Source: CAD feature listing. Evaluate the final solid. Frame: model axes, mm. Face numbers are marked on the shaded views. A direction names the side the tool comes from. Round coordinates to 2 decimals unless told otherwise and drop trailing zeros. Loops run counter-clockwise (first coordinate to the right, second up) from the corner with the lowest first, then second, coordinate; pieces in that order, holes last.
(1) Section D-D, the plane x = 241.3. Count the separate pieces of the cut face and the enclosed holes in it, plus the area to 3 significant figures.
(2) Section B-B, the plane x = 145.5. Return the cut outline in (y, z), plus the area to 3 significant figures.
(3) Section A-A, the plane z = 5.25. Return the cut outline in (x, y).
(4) Mould query, pull axis Y, two halves, no side actions, for the marked faces 3, 4 and 5. Classes: pulls with the +Y half, pulls with the -Y half, needs draft (parallel to the pull), parting line crosses it, or undercut.
(5) Section C-C, the plane y = 18.5. Return the cut outline in (x, z), plus the area to 3 significant figures.
(6) Material intervals for probe 1 along Y at (x, z) = (165.1, -12.25); probe 2 along Z at (x, y) = (114.3, -24.9); probe 3 along Y at (x, z) = (149.5, -2.5), sorted ascending.
(7) Set-up query: the marked faces 1 and 2. Return all of +Z, -Z, +X, -X, +Y, -Y with unobstructed straight access to the full face (end or side cutting, diameter ignored); none if empty.
```python
from build123d import *

# Parameters (mm, degrees)
F0_W     = 50.8
F0_H     = 25.4
F0_W_2   = 47.625
F0_H_2   = 22.225
F1_DEPTH = 254
F3_D     = 5.1054
F5_D     = 5.1054


with BuildPart() as f1:
    # F0 (on Right) → F1 (new body)
    with BuildSketch(Plane.YZ):
        Rectangle(F0_W, F0_H)
        Rectangle(F0_W_2, F0_H_2, mode=Mode.SUBTRACT)
    extrude(amount=F1_DEPTH)

    # F3 (through all)
    with Locations(Plane.XY.offset(12.7)):
        with Locations((38.1, -12.7), (63.5, 12.7), (63.5, -12.7), (88.9, 12.7), (88.9, -12.7), (114.3, 12.7), (241.3, -12.7), (215.9, -12.7), (190.5, -12.7), (165.1, -12.7), (241.3, 12.7), (215.9, 12.7), (114.3, -12.7), (190.5, 12.7), (139.7, 12.7), (139.7, -12.7), (165.1, 12.7), (12.7, 12.7), (12.7, -12.7), (38.1, 12.7)):
            Hole(F3_D / 2)

    # F5 (through all)
    with Locations(Plane(origin=(0, 25.4, 0), x_dir=(-1, 0, 0), z_dir=(0, 1, 0))):
        with Locations((-215.9, 0), (-165.1, 0), (-190.5, 0), (-139.7, 0), (-241.3, 0), (-114.3, 0), (-63.5, 0), (-88.9, 0), (-12.7, 0), (-38.1, 0)):
            Hole(F5_D / 2)


solid = f1.part
```
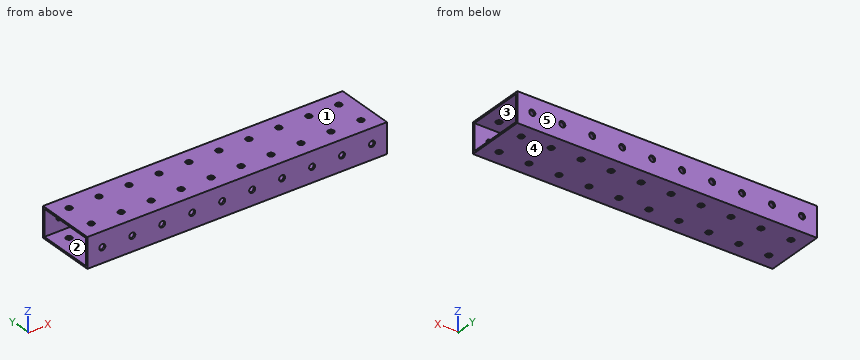
Output values:
1. separate pieces: 6
1. enclosed holes: 0
1. area: 183 mm2
2. outline: (-25.4, -12.7) - (25.4, -12.7) - (25.4, 12.7) - (-25.4, 12.7) - close; hole (-23.81, -11.11) - (23.81, -11.11) - (23.81, 11.11) - (-23.81, 11.11) - close
2. area: 232 mm2
3. outline: (0, -25.4) - (254, -25.4) - (254, -23.81) - (0, -23.81) - close; (0, 23.81) - (254, 23.81) - (254, 25.4) - (0, 25.4) - close
4. face 3: undercut
4. face 4: needs draft
4. face 5: pulls with the +Y half
5. outline: (0, -12.7) - (254, -12.7) - (254, -11.11) - (0, -11.11) - close; (0, 11.11) - (254, 11.11) - (254, 12.7) - (0, 12.7) - close
5. area: 806 mm2
6. probe 1: y = -25.4 to -15.25, -10.15 to 10.15, 15.25 to 25.4
6. probe 2: z = -12.7 to -2.55, 2.55 to 12.7
6. probe 3: y = -25.4 to -23.81, 23.81 to 25.4
7. face 1: +Z, +X, -X, +Y, -Y
7. face 2: +X, -X
